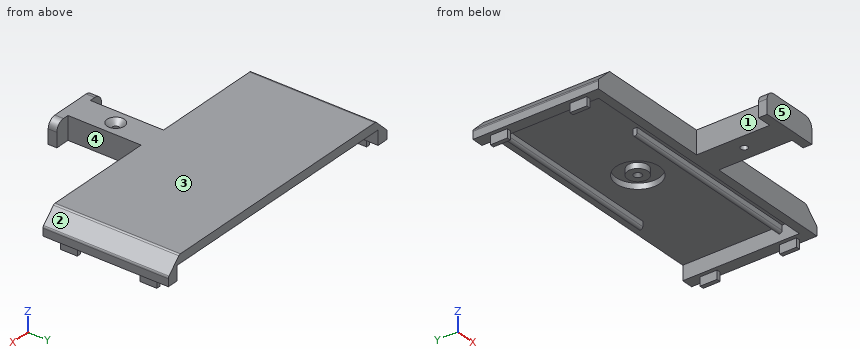
```python
from build123d import *

# Parameters (mm, degrees)
SKETCH2_W                                       = 96
SKETCH2_H                                       = 38.5
BOSS_EXTRUDE1_DEPTH                             = 3
BOSS_EXTRUDE2_DEPTH                             = 45
BOSS_EXTRUDE2_DEPTH_BACK                        = 20
BOSS_EXTRUDE3_DEPTH                             = 20
BOSS_EXTRUDE3_DEPTH_BACK                        = 45
SKETCH5_W                                       = 8
SKETCH5_H                                       = 5
BOSS_EXTRUDE4_DEPTH                             = 96
SKETCH6_W                                       = 3
SKETCH6_H                                       = 5
BOSS_EXTRUDE5_DEPTH                             = 38.5
SKETCH7_R                                       = 7.5
SKETCH7_R_2                                     = 3.5
CUT_EXTRUDE2_DEPTH                              = 2
MOVE_FACE1_BY                                   = 1
MOVE_FACE2_BY                                   = 1
SKETCH8_W                                       = 1.4
SKETCH8_H                                       = 5.9
BOSS_EXTRUDE6_DEPTH                             = 3
SKETCH9_W                                       = 10
SKETCH9_H                                       = 8
BOSS_EXTRUDE7_DEPTH                             = 25.4
SKETCH11_W                                      = 8
SKETCH11_H                                      = 3
BOSS_EXTRUDE8_DEPTH                             = 10
CHAMFER1_SIZE                                   = 5
FILLET1_R                                       = 1
FILLET3_R                                       = 3
MOVE_FACE3_BY                                   = 2
CSK_FOR_M2_FLAT_HEAD_MACHINE_SCREW1_D           = 2.4
CSK_FOR_M2_FLAT_HEAD_MACHINE_SCREW1_CSINK_D     = 6
CSK_FOR_M2_FLAT_HEAD_MACHINE_SCREW1_CSINK_ANGLE = 90


with BuildPart() as part:
    # Sketch2 → Boss-Extrude1 (new body)
    with BuildSketch(Plane.XY):
        Rectangle(SKETCH2_W, SKETCH2_H)
    extrude(amount=BOSS_EXTRUDE1_DEPTH)

    # Sketch3 → Boss-Extrude2 (add, two sides: drawn at the far end of the back side and taken through both)
    with BuildSketch(Plane(origin=(0, 0, 0), x_dir=(0, 0, -1), z_dir=(1, 0, 0)).offset(-BOSS_EXTRUDE2_DEPTH_BACK)):
        with BuildLine():
            Line((0, -15.25), (1.75, -15.25))
            ThreePointArc((1.75, -15.25), (2.5, -14.5), (1.75, -13.75))
            Line((1.75, -13.75), (0, -13.75))
            Line((0, -13.75), (0, -15.25))
        make_face()
    extrude(amount=BOSS_EXTRUDE2_DEPTH + BOSS_EXTRUDE2_DEPTH_BACK)

    # Sketch3<3> → Boss-Extrude3 (add, two sides: drawn at the far end of the back side and taken through both)
    with BuildSketch(Plane(origin=(0, 0, 0), x_dir=(0, 0, -1), z_dir=(1, 0, 0)).offset(-BOSS_EXTRUDE3_DEPTH_BACK)):
        with BuildLine():
            Line((0, 13.75), (0, 15.25))
            Line((0, 15.25), (1.75, 15.25))
            ThreePointArc((1.75, 15.25), (2.5, 14.5), (1.75, 13.75))
            Line((1.75, 13.75), (0, 13.75))
        make_face()
    extrude(amount=BOSS_EXTRUDE3_DEPTH + BOSS_EXTRUDE3_DEPTH_BACK)

    # Cut-Extrude1 cone 1 section (through the dimple's axis) → Cut-Extrude1 (revolve, cut)
    with BuildSketch(Plane.YZ):
        Polygon((0, 0), (1.375, 0), (0, 1.375), align=None)
    revolve(axis=Axis((0, 0, 0), (0, 0, 1)), mode=Mode.SUBTRACT)

    # Sketch5 → Boss-Extrude4 (add, through all)
    with BuildSketch(Plane.ZY.offset(48)):
        with Locations((-1, -21.75)):
            Rectangle(SKETCH5_W, SKETCH5_H)
    extrude(amount=-BOSS_EXTRUDE4_DEPTH)

    # Sketch6 → Boss-Extrude5 (add, through all)
    with BuildSketch(Plane(origin=(0, -19.25, 0), x_dir=(1, 0, 0), z_dir=(0, 1, 0))):
        with Locations((-46.5, 2.5)):
            Rectangle(SKETCH6_W, SKETCH6_H)
        with Locations((46.5, 2.5)):
            Rectangle(SKETCH6_W, SKETCH6_H)
    extrude(amount=BOSS_EXTRUDE5_DEPTH)

    # Sketch7 → Cut-Extrude2 (cut)
    with BuildSketch(Plane(origin=(0, 0, 0), x_dir=(-1, 0, 0), z_dir=(0, 0, -1))):
        Circle(SKETCH7_R)
        Circle(SKETCH7_R_2, mode=Mode.SUBTRACT)
    extrude(amount=-CUT_EXTRUDE2_DEPTH, mode=Mode.SUBTRACT)

    # Move Face1: a face moved outward by 1.0
    extrude(part.faces().sort_by_distance((-48, -2.5, -1))[0], amount=MOVE_FACE1_BY, dir=(-1, 0, 0))

    # Move Face2: a face moved outward by 1.0
    extrude(part.faces().sort_by_distance((48, -2.5, -1))[0], amount=MOVE_FACE2_BY, dir=(1, 0, 0))

    # Sketch8 → Boss-Extrude6 (add)
    with BuildSketch(Plane(origin=(0, 0, -5), x_dir=(-1, 0, 0), z_dir=(0, 0, -1))):
        with Locations((-47, 11.3)):
            Rectangle(SKETCH8_W, SKETCH8_H)
        with Locations((-47, -16.3)):
            Rectangle(SKETCH8_W, SKETCH8_H)
        with Locations((47, 11.3)):
            Rectangle(SKETCH8_W, SKETCH8_H)
        with Locations((47, -16.3)):
            Rectangle(SKETCH8_W, SKETCH8_H)
    extrude(amount=BOSS_EXTRUDE6_DEPTH)

    # Sketch9 → Boss-Extrude7 (add)
    with BuildSketch(Plane.XZ.offset(24.25)):
        with Locations((0, -1)):
            Rectangle(SKETCH9_W, SKETCH9_H)
    extrude(amount=BOSS_EXTRUDE7_DEPTH)

    # Sketch11 → Boss-Extrude8 (add, symmetric)
    with BuildSketch(Plane(origin=(0, 0, 0), x_dir=(0, 0, -1), z_dir=(1, 0, 0))):
        with Locations((1, -51.15)):
            Rectangle(SKETCH11_W, SKETCH11_H)
    extrude(amount=BOSS_EXTRUDE8_DEPTH, both=True)

    # Chamfer1
    chamfer1_edges = [part.edges().sort_by_distance(p)[0] for p in [
        (49, -2.5, 3),
        (-49, -2.5, 3),
    ]]
    chamfer(chamfer1_edges, length=CHAMFER1_SIZE)

    # Fillet1
    fillet1_edges = [part.edges().sort_by_distance(p)[0] for p in [
        (44, -2.5, 3),
        (-44, -2.5, 3),
        (-49, -2.5, -2),
        (49, -2.5, -2),
    ]]
    fillet(fillet1_edges, radius=FILLET1_R)

    # Fillet3
    fillet3_edges = [part.edges().sort_by_distance(p)[0] for p in [
        (-10, -51.15, 3),
        (10, -51.15, 3),
    ]]
    fillet(fillet3_edges, radius=FILLET3_R)

    # Move Face3: a face moved inward by 2.0
    extrude(part.faces().sort_by_distance((0, -19.25, -2.5))[0], amount=MOVE_FACE3_BY, dir=(0, -1, 0), mode=Mode.SUBTRACT)

    # CSK for M2 Flat Head Machine Screw1 (through all)
    with Locations(Plane.XY.offset(3)):
        with Locations((0, -36.95)):
            CounterSinkHole(CSK_FOR_M2_FLAT_HEAD_MACHINE_SCREW1_D / 2, CSK_FOR_M2_FLAT_HEAD_MACHINE_SCREW1_CSINK_D / 2, counter_sink_angle=CSK_FOR_M2_FLAT_HEAD_MACHINE_SCREW1_CSINK_ANGLE)


solid = part.part
```
The model under review builds one solid part; all positions refer to its coordinate system, in mm. Face numbers are marked on the shaded views. A direction names the side the tool comes from. Round coordinates to 2 decimals unless told otherwise and drop trailing zeros. Loops run counter-clockwise (first coordinate to the right, second up) from the corner with the lowest first, then second, coordinate; pieces in that order, holes last. Notation, with made-up numbers: (17.5, 80.5) - (65.5, 80.5) arc R30 cw to (65.5, 111.5) - close; hole circle Ø6 at (37.5, 44.25). An arc over 180 degrees is marked (long way). Use a Markdown table: item, result. Add a question column.
Q1. Add section D-D (y = -5). State the section outline as (x, z) points.
Q2. Add section A-A (y = -36.95). State the section outline as (x, z) points.
Q3. For probe 1 along Y at (x, z) = (0, -0.5); probe 2 along X at (y, z) = (7, -4.5); probe 3 along Y at (x, z) = (6, -3), list the stretches that pass through material, from the lowest coordinate up.
Q4. Machinability: for the marked faces 1 and 2, which of the approach directions +Z, -Z, +X, -X, +Y, -Y give a long, thin tool a straight path to every point of the face, cutting with its end or side? Answer none if there is none.
Q5. The part is to be moulded in two halves that separate along Y. For the marked faces 3, 4 and 5, say which applies: pulls with the +Y half, pulls with the -Y half, needs draft (parallel to the pull), parting line crosses it, or undercut.
Q6. Add section B-B (z = -3.5). State the section outline as (x, y) points, plus the area to 3 significant figures.
Q7. Add section C-C (x = -36). State the section outline as (y, z) points.
Q8. Insertion check: pin 1 Ø4 at (y, z) = (-41, 0.5) entering from +X; pin 2 Ø1 at (x, y) = (-16, -17) entering from -Z; pin 3 Ø0.9 at (x, z) = (12.5, -0.5) entering from +Y; pin 4 Ø6 at (x, y) = (23.5, -26) entering from +Z. Each pin has a flat end and moves straight along its axis. Give the tip position at first contact, or say it passes through.
Worked answers:
| question | item | result |
|---|---|---|
| 1 | outline | (-49, -5) - (-45, -5) - (-45, 0) - (-5.59, 0) - (-5.59, 2) - (5.59, 2) - (5.59, 0) - (45, 0) - (45, -5) - (49, -5) - (49, -2.41) arc R1 ccw to (48.71, -1.71) - (44.29, 2.71) arc R1 ccw to (43.59, 3) - (-43.59, 3) arc R1 ccw to (-44.29, 2.71) - (-48.71, -1.71) arc R1 ccw to (-49, -2.41) - close |
| 2 | outline | (-5, -5) - (-1.2, -5) - (-1.2, 1.2) - (-3, 3) - (-5, 3) - close; (1.2, -5) - (5, -5) - (5, 3) - (3, 3) - (1.2, 1.2) - close |
| 3 | probe 1 | -52.65 to -38.15, -35.75 to -21.25, -15.25 to -13.75, 13.75 to 15.25 |
| 3 | probe 2 | -49 to -45, 45 to 49 |
| 3 | probe 3 | -52.65 to -49.65, -24.25 to -21.25 |
| 4 | face 1 | +Z, -Z, -X |
| 4 | face 2 | +Z, +X, +Y, -Y |
| 5 | face 3 | needs draft |
| 5 | face 4 | undercut |
| 5 | face 5 | pulls with the -Y half |
| 6 | outline | (-49, -24.25) - (-5, -24.25) - (-5, -49.65) - (-10, -49.65) - (-10, -52.65) - (10, -52.65) - (10, -49.65) - (5, -49.65) - (5, -24.25) - (49, -24.25) - (49, 19.25) - (45, 19.25) - (45, -21.25) - (-45, -21.25) - (-45, 19.25) - (-49, 19.25) - close; hole circle Ø2.4 at (0, -36.95) |
| 6 | area | 927 mm² |
| 7 | outline | (-24.25, -5) - (-21.25, -5) - (-21.25, 0) - (13.75, 0) - (13.75, -1.75) arc R0.75 ccw to (15.25, -1.75) - (15.25, 0) - (19.25, 0) - (19.25, 3) - (-24.25, 3) - close |
| 8 | pin 1 | x = 5 |
| 8 | pin 2 | z = 0 |
| 8 | pin 3 | y = 15.25 |
| 8 | pin 4 | z = 3 |
